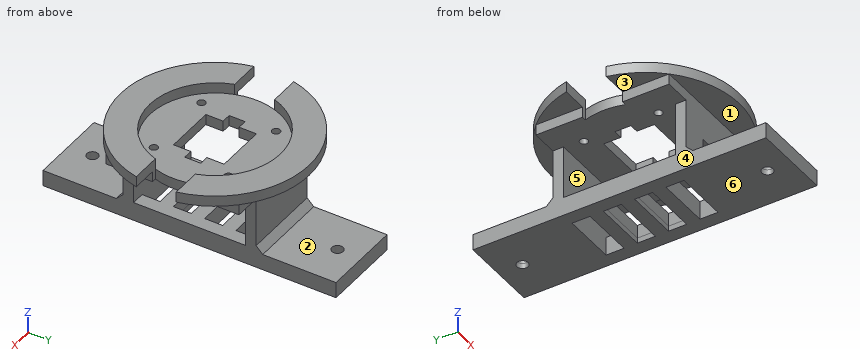
Autodesk Inventor part; units mm, degrees
ref_plane "YZ Plane" through (0, 0, 0) normal (1, 0, 0) x (0, 1, 0)
ref_plane "XZ Plane" through (0, 0, 0) normal (0, 1, 0) x (-1, 0, 0)
ref_plane "XY Plane" through (0, 0, 0) normal (0, 0, 1) x (1, 0, 0)
ref_plane "Arbeitsebene2" through (0, 0, 0) normal (0, 0, 1) x (1, 0, 0)
ref_plane "Arbeitsebene1" through (0, 0, -5) normal (0, 0, 1) x (1, 0, 0)
sketch "Skizze2" plane through (0, 0, 0) normal (0, 0, 1) x (1, 0, 0)
  line L0 (13.6, 12.5) -> (15, 12.5)
  arc A0 (10.4, 12.5) -> (13.6, 12.5) centre (12, 12.5) ccw
  line L1 (-10.4, 12.5) -> (10.4, 12.5)
  arc A1 (-13.6, 12.5) -> (-10.4, 12.5) centre (-12, 12.5) ccw
  line L2 (-15, 12.5) -> (-13.6, 12.5)
  line L3 (-15, 12.5) -> (-15, -12.5)
  line L4 (-15, -12.5) -> (-13.6, -12.5)
  arc A2 (-10.4, -12.5) -> (-13.6, -12.5) centre (-12, -12.5) ccw
  line L5 (-10.4, -12.5) -> (10.4, -12.5)
  arc A3 (13.6, -12.5) -> (10.4, -12.5) centre (12, -12.5) ccw
  line L6 (13.6, -12.5) -> (15, -12.5)
  line L7 (15, 12.5) -> (15, -12.5)
  line L8 (-8.2, 2) -> (-9, 2)
  arc A4 (-8.2, 2) -> (-8, 2.2) centre (-8.2, 2.2) ccw
  line L9 (-8, 7.8) -> (-8, 2.2)
  arc A5 (-7.8, 8) -> (-8, 7.8) centre (-7.8, 7.8) ccw
  line L10 (7.8, 8) -> (-7.8, 8)
  arc A6 (8, 7.8) -> (7.8, 8) centre (7.8, 7.8) ccw
  line L11 (8, 2.2) -> (8, 7.8)
  arc A7 (8, 2.2) -> (8.2, 2) centre (8.2, 2.2) ccw
  line L12 (9, 2) -> (8.2, 2)
  arc A8 (9, -2) -> (9, 2) centre (9, 0) ccw
  line L13 (8.2, -2) -> (9, -2)
  arc A9 (8.2, -2) -> (8, -2.2) centre (8.2, -2.2) ccw
  line L14 (8, -7.8) -> (8, -2.2)
  arc A10 (7.8, -8) -> (8, -7.8) centre (7.8, -7.8) ccw
  line L15 (-7.8, -8) -> (7.8, -8)
  arc A11 (-8, -7.8) -> (-7.8, -8) centre (-7.8, -7.8) ccw
  line L16 (-8, -2.2) -> (-8, -7.8)
  arc A12 (-8, -2.2) -> (-8.2, -2) centre (-8.2, -2.2) ccw
  line L17 (-9, -2) -> (-8.2, -2)
  arc A13 (-9, 2) -> (-9, -2) centre (-9, 0) ccw
  line L18 (-25, 25) -> (25, 25)
  line L19 (25, 25) -> (25, -25)
  line L20 (25, -25) -> (-25, -25)
  line L21 (-25, -25) -> (-25, 25)
  line L22 (0, 0) -> (0, -14)
  line L23 (0, -14) -> (14, -14)
  line L24 (14, -14) -> (14, 14)
  line L25 (14, 14) -> (-14, 14)
  line L26 (-14, 14) -> (-14, -14)
  circle A14 centre (14, -14) radius 1.5
  circle A15 centre (-14, -14) radius 1.5
  circle A16 centre (-14, 14) radius 1.5
  circle A17 centre (14, 14) radius 1.5
  dimension "d62" = 14
  dimension "d63" = 14
  dimension "d64" = 28
  dimension "d65" = 28
  dimension "d66" = 28
  dimension "d67" = 3
  dimension "d68" = 3
  dimension "d69" = 3
  dimension "d70" = 3
extrude "Extrusion1" add sketch "Skizze2" along normal blind 4 contours A0 L1 A1 L2 A16 L25 A17 L0 | L0 L24 L6 A3 L5 A2 L4 L26 L2 A1 L1 A0 | A15 | L0 L7 L6 L24 | A17 L25 L24 | L24 L25 A17 | A14 L23 L22 L5 A3 L6 | A14 L23 L24 | L24 L23 A14 | A16 L26 L25 | L25 L26 A16 | L26 L4 L3 L2 | L18 L19 L20 L21
sketch "Skizze3" plane through (0, 0, 4) normal (0, 0, 1) x (1, 0, 0)
  circle A0 centre (0, 0) radius 35.3553
  circle A1 centre (0, 0) radius 24.5
  point P0 (0, 0)
  dimension "d3" = 49
extrude "Extrusion2" add sketch "Skizze3" along normal blind 4
sketch "Skizze4" plane through (0, 0, 0) normal (0, 0, -1) x (-1, 0, 0)
  circle A0 centre (0, 0) radius 35.3553
  line L0 (25, 25) -> (25, -25)
  line L1 (-25, 25) -> (25, 25)
  line L2 (25, 25) -> (25, 21)
  line L3 (25, 21) -> (-25, 21)
  line L4 (-25, 21) -> (-25, 25)
  line L5 (-25, 25) -> (0, 25)
  line L6 (-25, 25) -> (25, 25)
  line L7 (0, 25) -> (15, 25)
  line L8 (15, 25) -> (-15, 25)
  line L9 (-15, 25) -> (-15, 21)
  line L10 (15, 25) -> (15, 21)
  line L11 (-15, 21) -> (15, 21)
  line L12 (-35.3553, 0) -> (35.3553, 0)
  line L13 (-15, -25) -> (-15, -21)
  line L14 (15, -25) -> (15, -21)
  line L15 (-15, -21) -> (15, -21)
  line L16 (15, -25) -> (-15, -25)
  line L17 (25, -25) -> (-25, -25)
  line L18 (15, 25) -> (-15, 25)
  point P0 (0, 0)
  dimension "d6" = 4
  dimension "d7" = 15
  dimension "d8" = 30
extrude "Extrusion3" add sketch "Skizze4" along normal blind 25 contours L10 L3 L9 L1 | L16 L13 L15 L14
sketch "Skizze5" plane through (-25, 25, 4) normal (0, 1, 0) x (1, 0, 0)
  line L0 (10, 29) -> (40, 29)
  line L1 (10, 4) -> (10, 29)
  line L2 (40, 29) -> (10, 29)
  line L3 (10, 29) -> (10, 25)
  line L4 (10, 25) -> (40, 25)
  line L5 (40, 25) -> (40, 29)
  line L6 (40, 29) -> (10, 29)
  line L7 (10, 4) -> (10, 29)
  point P0 (25, 4)
  dimension "d11" = 4
sketch "Skizze6" plane through (-25, -25, 4) normal (0, -1, 0) x (1, 0, 0)
  line L0 (10, -29) -> (40, -29)
  line L1 (10, -4) -> (10, -29)
  line L2 (40, -29) -> (10, -29)
  line L3 (10, -29) -> (10, -25)
  line L4 (10, -25) -> (40, -25)
  line L5 (40, -25) -> (40, -29)
  point P0 (25, -4)
  dimension "d12" = 4
extrude "Extrusion4" add sketch "Skizze6" along normal blind 30
extrude "Extrusion5" add sketch "Skizze5" along normal blind 30
sketch "Skizze7" plane through (-15, -21, 0) normal (0, 1, 0) x (1, 0, 0)
  line L0 (0, 25) -> (30, 25)
  line L1 (0, 0) -> (0, 25)
  line L2 (30, 0) -> (30, 25)
  line L3 (0, 25) -> (5, 25)
  line L4 (5, 25) -> (5, 20)
  line L5 (5, 20) -> (0, 20)
  line L6 (0, 20) -> (0, 25)
  line L7 (30, 25) -> (25, 25)
  line L8 (25, 25) -> (25, 20)
  line L9 (25, 20) -> (30, 20)
  line L10 (30, 20) -> (30, 25)
  point P0 (15, 0)
  point P1 (30, 20)
  point P2 (0, 20)
  point P3 (5, 25)
  dimension "d17" = 5
  dimension "d18" = 5
  dimension "d19" = 5
  dimension "d20" = 5
extrude "Extrusion6" add sketch "Skizze7" along normal blind 44
sketch "Skizze8" plane through (0, 0, 4) normal (0, 0, 1) x (1, 0, 0)
  line L0 (-9.5, 9.5) -> (-9.5, -9.5)
  line L1 (-9.5, -9.5) -> (9.5, -9.5)
  line L2 (9.5, -9.5) -> (9.5, 9.5)
  line L3 (9.5, 9.5) -> (-9.5, 9.5)
  line L4 (-9.5, 9.5) -> (-9.5, -9.5)
  line L5 (-5, -3) -> (-5, 3)
  line L6 (-5, -3) -> (-13, -3)
  line L7 (-13, -3) -> (-13, 3)
  line L8 (-13, 3) -> (-5, 3)
  line L9 (-5, 3) -> (-5, -3)
  line L10 (5.06, -3) -> (13.06, -3)
  line L11 (13.06, -3) -> (13.06, 3)
  line L12 (13.06, 3) -> (5.06, 3)
  line L13 (5.06, 3) -> (5.06, -3)
  point P0 (0, 0)
  point P1 (-9.5, -3)
  point P2 (9.5, -3)
  point P3 (9.5, 3)
  point P4 (-9.5, 3)
  dimension "d23" = 19
  dimension "d24" = 8
  dimension "d25" = 8
extrude "Extrusion7" cut sketch "Skizze8" against normal blind 15
chamfer "Fasen1" distance 2.5 angle 45 1 edges at (0, -25, -21)
chamfer "Fasen2" distance 2.5 angle 45 1 edges at (0, 25, -21)
sketch "Skizze11" plane through (-25, -25, 4) normal (0, -1, 0) x (1, 0, 0)
  line L0 (10, -4) -> (10, -22.5)
  line L1 (40, -22.5) -> (10, -22.5)
  line L2 (40, -4) -> (40, -22.5)
  line L3 (40, -4) -> (50, -4)
  line L4 (50, -4) -> (50, 0)
  line L5 (0, 0) -> (50, 0)
  line L6 (0, -4) -> (0, 0)
  line L7 (0, -4) -> (10, -4)
  line L8 (10, -4) -> (10, -22.5)
  line L9 (40, -22.5) -> (10, -22.5)
  line L10 (40, -4) -> (40, -22.5)
  line L11 (10, -22.5) -> (10, -25)
  line L12 (10, -22.5) -> (40, -22.5)
  line L13 (10, -22.5) -> (40, -22.5)
  line L14 (25, -22.5) -> (25, -19.5)
  line L15 (25, -19.5) -> (25, -16.5)
  line L16 (30, -19.75) -> (20, -19.75)
  line L17 (20, -19.75) -> (20, -13.25)
  line L18 (20, -13.25) -> (30, -13.25)
  line L19 (30, -13.25) -> (30, -19.75)
  line L20 (30, -19.75) -> (20, -13.25) construction
  line L21 (20, -19.75) -> (30, -13.25) construction
  point P0 (25, -4)
  point P1 (20.0696, -16.3928)
  dimension "d40" = 3
  dimension "d41" = 3
  dimension "d42" = 10
extrude "Extrusion10" cut sketch "Skizze11" against normal blind 8 contours L16 L17 L18 L19
sketch "Skizze12" plane through (-25, -25, 4) normal (0, -1, 0) x (1, 0, 0)
  line L0 (20, -13.25) -> (30, -13.25)
  line L1 (30, -13.25) -> (30, -19.75)
  line L2 (30, -19.75) -> (20, -19.75)
  line L3 (20, -19.75) -> (20, -13.25)
  line L4 (40, -22.5) -> (10, -22.5)
  line L5 (40, -4) -> (40, -22.5)
  line L6 (40, -4) -> (50, -4)
  line L7 (50, -4) -> (50, 0)
  line L8 (0, 0) -> (50, 0)
  line L9 (0, -4) -> (0, 0)
  line L10 (0, -4) -> (10, -4)
  line L11 (10, -4) -> (10, -22.5)
  line L12 (20.0696, -16.3928) -> (29.9304, -16.3928)
  line L13 (20, -19.75) -> (29.9304, -19.75)
  line L14 (29.9304, -19.75) -> (29.9304, -20.75)
  line L15 (29.9304, -20.75) -> (20, -20.75)
  line L16 (20, -20.75) -> (20, -19.75)
  point P0 (25, -4)
  dimension "d45" = 1
extrude "Extrusion11" cut sketch "Skizze12" against normal blind 7.25 contours L2 L14 L15 L16
sketch "Skizze13" plane through (0, 0, 8) normal (0, 0, 1) x (1, 0, 0)
  circle A0 centre (0, 0) radius 35.3553
  circle A1 centre (0, 0) radius 24.5
  circle A2 centre (0, 0) radius 24.5
  line L0 (-24.5, 0) -> (-36.4173, 0)
  arc A3 (-25, 25) -> (-25, -25) centre (0, 0) ccw
  line L1 (-35.3553, 0) -> (-35.3553, 7.5)
  line L2 (-35.3553, 7.5) -> (-23.3238, 7.5)
  line L3 (-35.3553, 0) -> (-35.3553, -7.5)
  line L4 (-35.3553, -7.5) -> (-23.3238, -7.5)
  circle A4 centre (0, 0) radius 35.3553
  line L5 (0, 35.3553) -> (0, -35.3553)
  line L6 (35.3553, 0) -> (35.3553, 7.5)
  line L7 (35.3553, 7.5) -> (23.3238, 7.5)
  line L8 (35.3553, 0) -> (35.3553, -7.5)
  line L9 (35.3553, -7.5) -> (23.3238, -7.5)
  point P0 (0, 0)
  point P1 (34.5507, -7.5)
  point P2 (34.5507, 7.5)
  point P3 (-34.5507, 7.5)
  point P4 (-34.5507, -7.5)
  dimension "d48" = 7.5
  dimension "d49" = 7.5
extrude "Extrusion12" cut sketch "Skizze13" against normal blind 47.75 contours A0 L9 A1 L7 | L2 A1 L0 A0 | L0 A1 L4 A0
sketch "Skizze14" plane through (-10, -21, -20) normal (1, 0, 0) x (0, 0, -1)
  line L0 (0, 42) -> (5, 42)
  line L1 (0, 0) -> (0, 42)
  line L2 (5, 0) -> (0, 0)
  line L3 (5, 0) -> (5, 42)
  line L4 (5, 42) -> (5, 21)
  line L5 (5, 21) -> (0, 21)
  line L6 (0, 0) -> (0, 42)
  line L7 (5, 21) -> (5, 18.5)
  line L8 (5, 0) -> (5, 42)
  line L9 (5, 18.5) -> (0, 18.5)
  line L10 (0, 18.5) -> (0, 23.5)
  line L11 (0, 23.5) -> (5, 23.5)
  line L12 (5, 23.5) -> (5, 18.5)
  point P0 (-20, 21)
  point P1 (0, 18.5)
  point P2 (5, 18.5)
  dimension "d52" = 2.5
  dimension "d53" = 5
extrude "Extrusion13" add sketch "Skizze14" along normal blind 21.25 contours L11 L3 L5 L1 | L5 L3 L9 L1
sketch "Skizze15" plane through (-15, -55, -21) normal (0, 0, 1) x (1, 0, 0)
  line L0 (0, 27.5) -> (30, 27.5)
  line L1 (0, 27.5) -> (0, 0)
  line L2 (30, 0) -> (0, 0)
  line L3 (30, 27.5) -> (30, 0)
  line L4 (30, 82.5) -> (0, 82.5)
  line L5 (30, 82.5) -> (30, 110)
  line L6 (0, 110) -> (30, 110)
  line L7 (0, 82.5) -> (0, 110)
  line L8 (15, 0) -> (15, 9)
  circle A0 centre (15, 9) radius 2.1
  line L9 (15, 110) -> (15, 101)
  circle A1 centre (15, 101) radius 2.1
  point P0 (15, 55)
  dimension "d56" = 9
  dimension "d57" = 4.2
  dimension "d58" = 9
  dimension "d59" = 4.2
extrude "Extrusion14" cut sketch "Skizze15" against normal blind 41.25 contours A0 | A1
sketch "Skizze16" plane through (0, 0, 4) normal (0, 0, 1) x (1, 0, 0)
  line L0 (0, 0) -> (0, -14)
  line L1 (0, -14) -> (14, -14)
  line L2 (14, -14) -> (-14, -14)
  line L3 (-14, -14) -> (-14, 14)
  line L4 (-14, 14) -> (14, 14)
  line L5 (14, 14) -> (14, -14)
  circle A0 centre (-14, -14) radius 1.5
  circle A1 centre (-14, 14) radius 1.5
  circle A2 centre (14, 14) radius 1.5
  circle A3 centre (14, -14) radius 1.5
  dimension "d71" = 14
  dimension "d72" = 14
  dimension "d73" = 28
  dimension "d74" = 28
  dimension "d75" = 3
  dimension "d76" = 3
  dimension "d77" = 3
  dimension "d78" = 3
extrude "Extrusion15" cut sketch "Skizze16" against normal blind 7.25 contours A3 L5 L1 | L1 L5 A3 | A0 L3 L2 | L2 L3 A0 | A2 L4 L5 | L5 L4 A2 | A1 L4 L3 | L3 L4 A1
sketch "Skizze17" plane through (-10, -21, -20) normal (1, 0, 0) x (0, 0, -1)
  point P0 (-20, 21)
sketch "Skizze18" plane through (-10, -21, -20) normal (1, 0, 0) x (0, 0, -1)
  line L0 (5, 18.5) -> (0, 18.5)
  line L1 (0, 0) -> (0, 18.5)
  line L2 (5, 0) -> (0, 0)
  line L3 (5, 0) -> (5, 18.5)
  line L4 (0, 23.5) -> (5, 23.5)
  line L5 (5, 23.5) -> (5, 42)
  line L6 (0, 42) -> (5, 42)
  line L7 (0, 23.5) -> (0, 42)
  line L8 (0, 0) -> (0, 9.25)
  line L9 (0, 0) -> (0, 18.5)
  line L10 (0, 0) -> (0, 42)
  line L11 (0, 32.75) -> (0, 30.25)
  line L12 (0, 9.25) -> (0, 6.75)
  line L13 (5, 42) -> (5, -34)
  line L14 (0, 6.75) -> (5, 6.75)
  line L15 (5, 6.75) -> (5, 11.75)
  line L16 (5, 11.75) -> (0, 11.75)
  line L17 (0, 11.75) -> (0, 6.75)
  line L18 (0, 30.25) -> (5, 30.25)
  line L19 (5, 30.25) -> (5, 35.25)
  line L20 (5, 35.25) -> (0, 35.25)
  line L21 (0, 35.25) -> (0, 30.25)
  point P0 (-20, 21)
  point P1 (0, 35.25)
  point P2 (0, 30.25)
  point P3 (0, 6.75)
  point P4 (5, 6.75)
  dimension "d81" = 2.5
  dimension "d82" = 2.5
  dimension "d83" = 5
  dimension "d84" = 5
extrude "Extrusion16" add sketch "Skizze18" along normal blind 23.25 contours L3 L14 L1 L16 | L18 L7 L20 L5
sketch "Skizze19" plane through (0, 0, -25) normal (0, 0, -1) x (-1, 0, 0)
  line L0 (10, 2.5) -> (10, 9.25)
  line L1 (10, 2.5) -> (-10, 2.5)
  line L2 (-10, 2.5) -> (-10, 9.25)
  line L3 (10, 9.25) -> (-10, 9.25)
  line L4 (10, -21) -> (10, -14.25)
  line L5 (10, -21) -> (-10, -21)
  line L6 (-10, -21) -> (-10, -14.25)
  line L7 (10, -14.25) -> (-10, -14.25)
  circle A0 centre (0, 46) radius 2.1
  circle A1 centre (0, -46) radius 2.1
  line L8 (10, -9.25) -> (-10, -9.25)
  line L9 (-10, -9.25) -> (-10, -2.5)
  line L10 (10, -2.5) -> (-10, -2.5)
  line L11 (10, -9.25) -> (10, -2.5)
  line L12 (10, 14.25) -> (-10, 14.25)
  line L13 (-10, 14.25) -> (-10, 21)
  line L14 (-10, 21) -> (10, 21)
  line L15 (10, 14.25) -> (10, 21)
  line L16 (-15, -55) -> (-15, 55)
  line L17 (15, -55) -> (-15, -55)
  line L18 (15, 21) -> (15, -55)
  line L19 (15, 21) -> (15, 55)
  line L20 (-15, 55) -> (15, 55)
  point P0 (0, 0)
extrude "Extrusion17" add sketch "Skizze19" along normal blind 2
properties part number "CAM1"
Model file for the job. Use its own axes, mm. Face numbers are marked on the shaded views. A direction names the side the tool comes from. Round coordinates to 2 decimals unless told otherwise and drop trailing zeros. Loops run counter-clockwise (first coordinate to the right, second up) from the corner with the lowest first, then second, coordinate; pieces in that order, holes last. Notation, with made-up numbers: M 74,87.5 L 112,87.5 A12 ccw 112,106.5 Z; hole C 0,-37.75 d11. An arc over 180 degrees is marked long. Put each result on its own line as item: value. Start each with the question number.
Item 1: Cut at A-A (y = 46). List the corners of the cut face in (x, z), then the cut area to 3 significant figures.
Item 2: Mould opens along Z. For the marked faces 4, 5 and 6 say: released by +Z, released by -Z, zero draft, split by the parting line, or undercut.
Item 3: Cut at C-C (y = -18.5). List the corners of the cut face in (x, z).
Item 4: 3-axis set-ups, long thin cutter, end or side, ignore diameter. For the marked faces 1, 2 and 3: which of +Z, -Z, +X, -X, +Y, -Y reach the whole face in a straight line?
Item 5: Drop flat-ended pins along their axis: P1, Ø3.5, axis at y = 17.5, z = -24, coming from the +X side; P2, Ø6, axis at y = -0.5, z = 1.5, coming from the +X side; P3, Ø4.5, axis at y = -19.5, z = 1, coming from the +X side. Give the stop position or say it passes through.
Item 6: Drill centre lines: line 1 along X through (y, z) = (14, 2); line 2 along Y through (x, z) = (13, -13.5). Where is each one in solid material? Low to high.
Item 7: Cut at B-B (z = -3). List the corners of the cut face in (x, y).
Item 8: Cut at D-D (z = -23). List the corners of the cut face in (x, y), then the cut area to 3 significant figures.
Answer block:
1. outline: M -15,-27 L -2.1,-27 L -2.1,-21 L -15,-21 Z; M 2.1,-27 L 15,-27 L 15,-21 L 2.1,-21 Z
1. area: 155 mm2
2. face 4: zero draft
2. face 5: undercut
2. face 6: released by -Z
3. outline: M -30.13,4 L -25,4 L -25,0 L 25,0 L 25,4 L 30.13,4 L 30.13,8 L 16.06,8 L 16.06,4 L -16.06,4 L -16.06,8 L -30.13,8 Z; M -15,-27 L -10,-27 L -10,-20 L -15,-20 Z; M 10,-27 L 15,-27 L 15,-20 L 10,-20 Z
4. face 1: +X, -X, -Y
4. face 2: +X, -X, +Y
4. face 3: -Z, -X, +Y, -Y
5. P1: x = 15
5. P2: x = 24.5
5. P3: x = 25
6. line 1: -25 to -15.5, -12.5 to 12.5, 15.5 to 25
6. line 2: -25 to -21, 21 to 25
7. outline: M -15,-25 L 15,-25 L 15,-21 L -15,-21 Z; M -15,21 L 15,21 L 15,25 L -15,25 Z
8. outline: M -15,-55 L 15,-55 L 15,55 L -15,55 Z; hole M -10,-21 L 10,-21 L 10,-14.25 L -10,-14.25 Z; hole M -10,-9.25 L 10,-9.25 L 10,-2.5 L -10,-2.5 Z; hole M -10,2.5 L 10,2.5 L 10,9.25 L -10,9.25 Z; hole M -10,14.25 L 10,14.25 L 10,21 L -10,21 Z; hole C 0,-46 d4.2; hole C 0,46 d4.2
8. area: 2,730 mm2
